```python
from build123d import *

# Parameters (mm, degrees)
F0_R     = 1.905
F0_R_2   = 3.175
F1_DEPTH = 3.175
F0_R_3   = 2.1456580426
F2_DEPTH = 6.35


# Not quite as in the source:
# - ends of sketch curves that miss each other by under 0.0002 mm in the source are joined


with BuildPart() as f1:
    # F0 (on Top) → F1 (new body)
    with BuildSketch(Plane.XY):
        Polygon((44.45, 44.4739684463), (-44.45, 44.4739684463), (-44.45, -126.9760241032), (44.4500006139, -126.9760241032), align=None)
        with Locations((-35.7399480417, -119.4167938083)):
            Circle(F0_R, mode=Mode.SUBTRACT)
        with Locations((-35.7399480417, -47.9368977249)):
            Circle(F0_R, mode=Mode.SUBTRACT)
        with Locations((-24.13, -60.7800519583)):
            Circle(F0_R_2, mode=Mode.SUBTRACT)
        Polygon((-16.5099999687, 14.3167711779), (-16.5099999992, 20.6667711779), (16.5100000008, 20.6667711779), (16.5100000313, 14.3167711779), (36.0137783311, 14.3167711779), (36.0137783311, -29.7200025995), (16.5100000008, -29.7200026932), (16.5099995171, -65.6599379314), (36.013777817, -65.6599379314), (36.013777817, -109.6967117089), (16.5099994866, -109.6967118025), (16.5099995476, -116.0467118025), (-16.5100004524, -116.0467118025), (-16.5100004829, -109.6967118025), (-36.0137786019, -109.6967118961), (-36.0137788132, -65.659938025), (-16.5100004829, -65.6599379314), (-16.5099999687, -29.7200026932), (-36.0137780877, -29.7200027868), (-36.0137782991, 14.3167710843), align=None, mode=Mode.SUBTRACT)
        with Locations((35.7399480417, -119.4167938083)):
            Circle(F0_R, mode=Mode.SUBTRACT)
        with Locations((24.1312399077, -54.422124289)):
            Circle(F0_R_2, mode=Mode.SUBTRACT)
        with Locations((35.7399480417, -47.9368977249)):
            Circle(F0_R, mode=Mode.SUBTRACT)
        with Locations((-35.7399480417, -35.6178977249)):
            Circle(F0_R, mode=Mode.SUBTRACT)
        with Locations((-24.142025454, 21.7699480417)):
            Circle(F0_R_2, mode=Mode.SUBTRACT)
        with Locations((-35.7399480417, 35.7399480417)):
            Circle(F0_R, mode=Mode.SUBTRACT)
        with Locations((35.7399480417, -35.7399480417)):
            Circle(F0_R, mode=Mode.SUBTRACT)
        with Locations((24.13, 20.4999480417)):
            Circle(F0_R_2, mode=Mode.SUBTRACT)
        with Locations((35.7399480417, 35.7399480417)):
            Circle(F0_R, mode=Mode.SUBTRACT)
    extrude(amount=F1_DEPTH)

    # F0 (on Top) → F2 (join)
    with BuildSketch(Plane.XY):
        with Locations((-24.13, -60.7800519583)):
            Circle(F0_R_2)
        with Locations((-24.13, -60.7800519583)):
            Circle(F0_R_3, mode=Mode.SUBTRACT)
        with Locations((-24.142025454, 21.7699480417)):
            Circle(F0_R_2)
        with Locations((-24.142025454, 21.7699480417)):
            Circle(F0_R_3, mode=Mode.SUBTRACT)
        with Locations((24.1312399077, -54.422124289)):
            Circle(F0_R_2)
        with Locations((24.1312399077, -54.422124289)):
            Circle(F0_R_3, mode=Mode.SUBTRACT)
        with Locations((24.13, 20.4999480417)):
            Circle(F0_R_2)
        with Locations((24.13, 20.4999480417)):
            Circle(F0_R_3, mode=Mode.SUBTRACT)
    extrude(amount=F2_DEPTH)


solid = f1.part
```
Input: part model. Units: mm. Frame: model coordinates. A direction names the side the tool comes from. Coordinates: 2 decimals unless noted, no trailing zeros. Write each loop counter-clockwise with the first axis right and the second up, starting at its lowest first coordinate (ties: lowest second). Pieces come first, ordered by that corner, then holes. Notation, with made-up numbers: M 64,-11 L 88,-11 A26 ccw 88,27 Z; hole C 68,26 d5. An arc over 180 degrees is marked long. Use one line per item in the form item = value.
Q1. Section D-D (z = 2). Count the separate pieces of the cut face and the enclosed holes in it, plus the area to 3 significant figures.
Answer below:
separate_pieces = 1
enclosed_holes = 13
area = 7,140 mm²
Q2. Material intervals for probe 1 along Y at (x, z) = (-19, 1); probe 2 along Y at (x, z) = (24.13, 2.5); probe 3 along X at (y, z) = (-33, 2), sorted ascending. Write a range as from..to.
Answer below:
probe_1 = -126.98..-109.7, -65.66..-29.72, 14.32..44.47
probe_2 = -126.98..-109.7, -65.66..-56.57, -52.28..-29.72, 14.32..18.35, 22.65..44.47
probe_3 = -44.45..-16.51, 16.51..44.45
Q3. Section A-A (x = 24.13). Return loops of the section in (y, z) (3 decimals).
Answer below:
outline = M -126.976,0 L -109.697,0 L -109.697,3.175 L -126.976,3.175 Z; M -65.66,0 L -56.568,0 L -56.568,6.35 L -57.597,6.35 L -57.597,3.175 L -65.66,3.175 Z; M -52.276,0 L -29.72,0 L -29.72,3.175 L -51.247,3.175 L -51.247,6.35 L -52.276,6.35 Z; M 14.317,0 L 18.354,0 L 18.354,6.35 L 17.325,6.35 L 17.325,3.175 L 14.317,3.175 Z; M 22.646,0 L 44.474,0 L 44.474,3.175 L 23.675,3.175 L 23.675,6.35 L 22.646,6.35 Z
Q4. Set-up query: faces 4 (the face through (36.014, -7, 2)), 5 (the face through (-1, -126.976, 2)), 6 (the face through (-21.21, 20.55, 4.74)). Return all of +Z, -Z, +X, -X, +Y, -Y with unobstructed straight access to the full face (end or side cutting, diameter ignored); none if empty.
Answer below:
face_4 = +Z, -Z
face_5 = +Z, -Z, +X, -X, -Y
face_6 = +Z
Q5. Section B-B (y = -99). Return loops of the section in (x, z) (3 decimals), plus the area to 3 significant figures.
Answer below:
outline = M -44.45,0 L -36.014,0 L -36.014,3.175 L -44.45,3.175 Z; M 36.014,0 L 44.45,0 L 44.45,3.175 L 36.014,3.175 Z
area = 53.6 mm²
Q6. Section C-C (x = 8). Return loops of the section in (y, z) (3 decimals), plus the area to 3 significant figures.
Answer below:
outline = M -126.976,0 L -116.047,0 L -116.047,3.175 L -126.976,3.175 Z; M 20.667,0 L 44.474,0 L 44.474,3.175 L 20.667,3.175 Z
area = 110 mm²
Q7. Draft query along X for faces 1 (the face through (44.45, -42, 2)), 2 (the face through (-20, -40, 0)), 3 (the face through (-16.51, 17, 2)). Return one class per face: released by +X, released by -X, zero draft, split by the parting line, or undercut.
Answer below:
face_1 = released by +X
face_2 = zero draft
face_3 = undercut
Q8. First-contact query: pin 1 (6 mm diameter, centred on x = -35.74, y = 35.74, fed in from +Z) (3 decimals). Flat tip, straight axial feed; report the tip coordinate or a pass-through.
Answer below:
pin_1 = 3.175
